```python
from build123d import *

# Parameters (mm, degrees)
F0_R        = 5.9508004686
F0_R_2      = 1.5
F1_DEPTH    = 3.175
F2_W        = 6.35
F2_H        = 6.35
F2_R        = 1.5
F3_DEPTH    = 6.35
F4_R        = 1.35255
F5_REACH    = 12.9523895761
F6_T1_DEPTH = 6.35
F8_DEPTH    = 3.175
F9_COUNT    = 12
F9_ANGLE    = 330


# Not quite as in the source:
# - a fillet or chamfer that OpenCascade refuses, or shapes differently, is made with other operations: its cross-section is extruded or revolved along the edge and cut away or added


with BuildPart() as f1:
    # F0 (on Top) → F1 (new body)
    with BuildSketch(Plane.XY):
        Circle(F0_R)
        Circle(F0_R_2, mode=Mode.SUBTRACT)
    extrude(amount=F1_DEPTH)

    # F2 (on face) → F3 (join)
    with BuildSketch(Plane.XY.offset(3.175)):
        Rectangle(F2_W, F2_H)
        Circle(F2_R, mode=Mode.SUBTRACT)
    extrude(amount=F3_DEPTH)

    f5_end = f1.faces().sort_by_distance((-1.5, 0, 4.7625))[0]
    # F4 (on face) → F5 (cut, up to a face of the model that its end follows)
    with BuildSketch(Plane.YZ.offset(3.175)):
        with Locations((0, 6.35)):
            Circle(F4_R)
    f5_long = extrude(amount=-F5_REACH, mode=Mode.PRIVATE)
    add(split(f5_long, bisect_by=f5_end, keep=Keep.ALL, mode=Mode.PRIVATE).solids().sort_by_distance((3.175, 0, 6.35))[0], mode=Mode.SUBTRACT)

    # F6: fillet of radius 3.175 on 4 edges, made by hand

    # F6_s2 → F6_t1 (cut)
    with BuildSketch(Plane.XY.offset(3.175)):
        with BuildLine():
            ThreePointArc((0, -3.175), (2.2450640303, -2.2450640303), (3.175, 0))
            Line((3.175, 0), (3.2385, 0))
            Line((3.2385, 0), (3.2385, -3.2385))
            Line((3.2385, -3.2385), (0, -3.2385))
            Line((0, -3.2385), (0, -3.175))
        make_face()
        with BuildLine():
            ThreePointArc((0, -3.175), (-2.2450640303, -2.2450640303), (-3.175, 0))
            Line((-3.175, 0), (-3.2385, 0))
            Line((-3.2385, 0), (-3.2385, -3.2385))
            Line((-3.2385, -3.2385), (0, -3.2385))
            Line((0, -3.2385), (0, -3.175))
        make_face()
        with BuildLine():
            ThreePointArc((3.175, 0), (2.2450640303, 2.2450640303), (0, 3.175))
            Line((0, 3.175), (0, 3.2385))
            Line((0, 3.2385), (3.2385, 3.2385))
            Line((3.2385, 3.2385), (3.2385, 0))
            Line((3.2385, 0), (3.175, 0))
        make_face()
        with BuildLine():
            ThreePointArc((0, 3.175), (-2.2450640303, 2.2450640303), (-3.175, 0))
            Line((-3.175, 0), (-3.2385, 0))
            Line((-3.2385, 0), (-3.2385, 3.2385))
            Line((-3.2385, 3.2385), (0, 3.2385))
            Line((0, 3.2385), (0, 3.175))
        make_face()
    extrude(amount=F6_T1_DEPTH, mode=Mode.SUBTRACT)

    # F7 (on face) → F8 (cut, through all)
    with BuildSketch(Plane(origin=(0, 0, 0), x_dir=(1, 0, 0), z_dir=(0, 0, -1))):
        with BuildLine():
            Line((4.0897477961, -0.2617496271), (5.8282529848, -1.2014546857))
            ThreePointArc((5.8282529848, -1.2014546857), (5.9508004686, 0), (5.8282529848, 1.2014546857))
            Line((5.8282529848, 1.2014546857), (4.0897477961, 0.2617496271))
            ThreePointArc((4.0897477961, 0.2617496271), (3.9336899209, 0), (4.0897477961, -0.2617496271))
        make_face()
    f8 = extrude(amount=-F8_DEPTH, mode=Mode.SUBTRACT)

    # F9: F8 ×12 about axis
    f9_axis = Axis((0, 0, 0), (0, 0, -1))
    for i in range(1, F9_COUNT):
        add(f8.rotate(f9_axis, i * F9_ANGLE / (F9_COUNT - 1)), mode=Mode.SUBTRACT)


solid = f1.part
```
Part model, mm, in its own coordinate system. A direction names the side the tool comes from. Coordinates: 2 decimals unless noted, no trailing zeros. Loops run counter-clockwise (first coordinate to the right, second up) from the corner with the lowest first, then second, coordinate; pieces in that order, holes last. Notation, with made-up numbers: (37, -19) - (58, -19) arc R21 ccw to (58, -10) - close; hole circle Ø9 at (-27, -15.75). An arc over 180 degrees is marked (long way). Write item = value, one per line. Start each with the question number.
Item 1: Cut at C-C, the plane y = -0.75. Give the cut face in (x, z) (3 decimals), and give its area (3 significant figures).
Item 2: Mould opens along Z. For faces 1 (the cylindrical face through (1.93, 1.25, 5.83)), 2 (the flat face through (1.2, -1.2, 0)), 3 (the flat face through (-0.7, 4.9, 1.6)) say: released by +Z, released by -Z, zero draft, split by the parting line, or undercut.
Item 3: Flat gauge pins, fed straight in: pin 1 Ø4.5 at (y, z) = (0, 6.35) entering from -X (3 decimals); pin 2 Ø1.5 at (x, z) = (-2.5, 7) entering from -Y; pin 3 Ø1 at (x, z) = (0, 3) entering from +Y; pin 4 Ø1.8 at (x, y) = (0, 0) entering from -Z. Where does each tip first touch, or does it go through?
Item 4: Cut at B-B, the plane z = 9.25. Give the cut face in (x, y) (3 decimals).
Item 5: Wall check: L1, parallel to Z at x = 2, y = 0 (3 decimals); L2, parallel to Y at x = 1.2, z = 6.35; L3, parallel to Z at x = -2.5, y = 2 (3 decimals). Give the ranges that are in metal, low to high. Write a range as from..to.
Item 6: Cut at A-A, the plane x = 4.75. Give the cut face in (y, z) (3 decimals), and give its area (3 significant figures).
Item 7: Cut at D-D, the plane y = 4.25. Give the cut face in (x, z) (3 decimals), and give its area (3 significant figures).
Item 8: 3-axis set-ups, long thin cutter, end or side, ignore diameter. For faces 4 (the flat face through (4.971, -0.738, 1.565)), 5 (the flat face through (0.7, 1.5, 9.525)), 6 (the flat face through (-0.738, -4.971, 1.565)), 7 (the flat face through (0.738, 4.971, 1.565)), 8 (the cylindrical face through (-1.5, 0.07, 4.7)): which of +Z, -Z, +X, -X, +Y, -Y reach the whole face in a straight line?
The answers:
q1.outline = (-4.993, 0) - (-1.299, 0) - (-1.299, 9.525) - (-3.085, 9.525) - (-3.085, 3.175) - (-4.993, 3.175) - close; (1.299, 0) - (4.993, 0) - (4.993, 3.175) - (3.085, 3.175) - (3.085, 5.224) - (1.299, 5.224) - close; (1.299, 7.476) - (3.085, 7.476) - (3.085, 9.525) - (1.299, 9.525) - close
q1.area = 42.1 mm2
q2.face_1 = undercut
q2.face_2 = released by -Z
q2.face_3 = zero draft
q3.pin_1 = -3.175
q3.pin_2 = -2.65
q3.pin_3 = 4.53
q3.pin_4 = through
q4.outline = circle Ø6.35 at (0, 0); hole circle Ø3 at (0, 0)
q5.L1 = 0..4.997, 7.703..9.525
q5.L2 = -2.94..-1.35, 1.35..2.94
q5.L3 = 0..3.175
q6.outline = (-1.848, 0) - (-0.619, 0) - (-0.619, 3.175) - (-1.848, 3.175) - close; (0.619, 0) - (1.848, 0) - (1.848, 3.175) - (0.619, 3.175) - close
q6.area = 7.81 mm2
q7.outline = (-4.165, 0) - (-3.635, 0) - (-3.635, 3.175) - (-4.165, 3.175) - close; (-1.834, 0) - (-0.348, 0) - (-0.348, 3.175) - (-1.834, 3.175) - close; (0.348, 0) - (1.834, 0) - (1.834, 3.175) - (0.348, 3.175) - close; (3.635, 0) - (4.165, 0) - (4.165, 3.175) - (3.635, 3.175) - close
q7.area = 12.8 mm2
q8.face_4 = +Z, -Z, +X
q8.face_5 = +Z, +X, -X, +Y, -Y
q8.face_6 = +Z, -Z, -Y
q8.face_7 = +Z, -Z, +Y
q8.face_8 = +Z, -Z
